from build123d import *

# Parameters (mm, degrees)
SKETCH_1_W               = 33.5
SKETCH_1_H               = 32
SKETCH_1_R               = 1.5
EXTRUDE_1_DEPTH          = 38
SKETCH_2_W               = 33
SKETCH_2_H               = 32
CUT_EXTRUDE_1_DEPTH      = 31
SKETCH_4_R               = 11.5
CUT_EXTRUDE_2_DEPTH      = 39
SKETCH_5_W               = 31
SKETCH_5_H               = 19
CUT_EXTRUDE_3_DEPTH      = 33.5
CUT_EXTRUDE_3_DEPTH_BACK = 11.5
SKETCH_8_W               = 38
SKETCH_8_H               = 32
EXTRUDE_3_DEPTH          = 4
EXTRUDE_4_DEPTH          = 9
SKETCH_11_W              = 8
SKETCH_11_H              = 1.5
CUT_EXTRUDE_4_DEPTH      = 10
FILLET_3_R               = 1
SKETCH_12_R              = 1.75
CUT_EXTRUDE_5_DEPTH      = 47.5
SKETCH_13_R              = 3.5
CUT_EXTRUDE_6_DEPTH      = 10
SKETCH_15_W              = 31.5
SKETCH_15_H              = 32
CUT_EXTRUDE_7_DEPTH      = 4
SKETCH_16_R              = 3
CUT_EXTRUDE_8_DEPTH      = 3
FILLET_4_R               = 5


with BuildPart() as part:
    # Эскиз1 → Бобышка-Вытянуть1 (new body)
    with BuildSketch(Plane.XY):
        with Locations((2.5, 0)):
            Rectangle(SKETCH_1_W, SKETCH_1_H)
        with Locations((10.25, -10)):
            Circle(SKETCH_1_R, mode=Mode.SUBTRACT)
        with Locations((-10.25, -10)):
            Circle(SKETCH_1_R, mode=Mode.SUBTRACT)
        with Locations((14.25, -10)):
            Circle(SKETCH_1_R, mode=Mode.SUBTRACT)
        with Locations((14.25, 10)):
            Circle(SKETCH_1_R, mode=Mode.SUBTRACT)
        with Locations((10.25, 10)):
            Circle(SKETCH_1_R, mode=Mode.SUBTRACT)
        with Locations((-10.25, 10)):
            Circle(SKETCH_1_R, mode=Mode.SUBTRACT)
    extrude(amount=-EXTRUDE_1_DEPTH)

    # Эскиз2 → Вырез-Вытянуть1 (cut)
    with BuildSketch(Plane.ZY.offset(14.25)):
        with Locations((-19, 0)):
            Rectangle(SKETCH_2_W, SKETCH_2_H)
    extrude(amount=-CUT_EXTRUDE_1_DEPTH, mode=Mode.SUBTRACT)

    # Эскиз4 → Вырез-Вытянуть2 (cut, through all)
    with BuildSketch(Plane(origin=(0, 0, -38), x_dir=(-1, 0, 0), z_dir=(0, 0, -1))):
        with Locations((19.35, 0)):
            Circle(SKETCH_4_R)
    extrude(amount=-CUT_EXTRUDE_2_DEPTH, mode=Mode.SUBTRACT)

    # Эскиз5 → Вырез-Вытянуть3 (cut, two sides)
    with BuildSketch(Plane.XY.offset(-35.5)) as cut_extrude_3_sk:
        with Locations((1.25, 0)):
            Rectangle(SKETCH_5_W, SKETCH_5_H)
    extrude(amount=CUT_EXTRUDE_3_DEPTH, mode=Mode.SUBTRACT)
    extrude(cut_extrude_3_sk.sketch, amount=-CUT_EXTRUDE_3_DEPTH_BACK, mode=Mode.SUBTRACT)

    # Эскиз8 → Бобышка-Вытянуть3 (add)
    with BuildSketch(Plane(origin=(19.25, 0, 0), x_dir=(0, 0, -1), z_dir=(1, 0, 0))):
        with Locations((19, 0)):
            Rectangle(SKETCH_8_W, SKETCH_8_H)
    extrude(amount=EXTRUDE_3_DEPTH)

    # Эскиз10 → Бобышка-Вытянуть4 (add)
    with BuildSketch(Plane(origin=(23.25, 0, 0), x_dir=(0, 0, -1), z_dir=(1, 0, 0))):
        with BuildLine():
            Line((38, 16), (0, 16))
            Line((0, 16), (-22.964648913, 10.720331419))
            ThreePointArc((-22.964648913, 10.720331419), (-31.5, 0), (-22.964648913, -10.720331419))
            Line((-22.964648913, -10.720331419), (0, -16))
            Line((0, -16), (38, -16))
            Line((38, -16), (38, 16))
        make_face()
    extrude(amount=EXTRUDE_4_DEPTH)

    # Эскиз11 → Вырез-Вытянуть4 (cut)
    with BuildSketch(Plane(origin=(0, 0, -38), x_dir=(-1, 0, 0), z_dir=(0, 0, -1))):
        with Locations((4.25, 10.25)):
            Rectangle(SKETCH_11_W, SKETCH_11_H)
        with Locations((4.25, -10.25)):
            Rectangle(SKETCH_11_W, SKETCH_11_H)
    extrude(amount=-CUT_EXTRUDE_4_DEPTH, mode=Mode.SUBTRACT)

    # Скругление3
    fillet_3_edges = [part.edges().sort_by_distance(p)[0] for p in [
        (-14.25, -16, -36.75),
        (-14.25, 16, -36.75),
        (-0.25, 11, -36.75),
        (-8.25, -11, -36.75),
        (-0.25, -11, -36.75),
        (-14.25, 16, -1.25),
        (-14.25, -16, -1.25),
        (-14.25, 10.307278981, -1.25),
        (-14.25, -10.307278981, -1.25),
        (-14.25, 10.307278981, -36.75),
        (-14.25, -10.307278981, -36.75),
    ]]
    fillet(fillet_3_edges, radius=FILLET_3_R)

    # Эскиз12 → Вырез-Вытянуть5 (cut, through all)
    with BuildSketch(Plane(origin=(32.25, 0, 0), x_dir=(0, 0, -1), z_dir=(1, 0, 0))):
        with Locations((-27.5, 0)):
            Circle(SKETCH_12_R)
        with Locations((-20.5, 7)):
            Circle(SKETCH_12_R)
        with Locations((-13.5, 0)):
            Circle(SKETCH_12_R)
        with Locations((-20.5, -7)):
            Circle(SKETCH_12_R)
    extrude(amount=-CUT_EXTRUDE_5_DEPTH, mode=Mode.SUBTRACT)

    # Эскиз13 → Вырез-Вытянуть6 (cut)
    with BuildSketch(Plane.ZY.offset(-23.25)):
        with Locations((20.5, 0)):
            Circle(SKETCH_13_R)
    extrude(amount=-CUT_EXTRUDE_6_DEPTH, mode=Mode.SUBTRACT)

    # Эскиз15 → Вырез-Вытянуть7 (cut)
    with BuildSketch(Plane.ZY.offset(-23.25)):
        with Locations((15.75, 0)):
            Rectangle(SKETCH_15_W, SKETCH_15_H)
    extrude(amount=-CUT_EXTRUDE_7_DEPTH, mode=Mode.SUBTRACT)

    # Эскиз16 → Вырез-Вытянуть8 (cut)
    with BuildSketch(Plane.ZY.offset(-27.25)):
        with Locations((20.5, 7)):
            Circle(SKETCH_16_R)
        with Locations((27.5, 0)):
            Circle(SKETCH_16_R)
        with Locations((20.5, -7)):
            Circle(SKETCH_16_R)
        with Locations((13.5, 0)):
            Circle(SKETCH_16_R)
    extrude(amount=-CUT_EXTRUDE_8_DEPTH, mode=Mode.SUBTRACT)

    # Скругление4
    fillet_4_edges = [part.edges().sort_by_distance(p)[0] for p in [
        (27.25, 0, 0),
    ]]
    fillet(fillet_4_edges, radius=FILLET_4_R)


solid = part.part
Read the model definition and answer for the solid it produces. Units are mm, in the model's axes. A direction names the side the tool comes from. Round coordinates to 2 decimals unless told otherwise and drop trailing zeros. Loops run counter-clockwise (first coordinate to the right, second up) from the corner with the lowest first, then second, coordinate; pieces in that order, holes last.
Q1. Determine the mould class of faces 1 (the face through (-7.85, 0.17, -0.99)), 2 (the face through (1, 13, -35.5)), 3 (the face through (14.2, -11.5, -36.7)) for opening direction X: released by +X, released by -X, zero draft, split by the parting line, or undercut.
Q2. Section A-A on x = 2.5 is taken. Write down the section's boundary in (y, z), and give its area (3 significant figures).
Q3. Each of these flat-tipped pins is pushed along its axis until it touches: pin 1 (2 mm diameter, centred on x = -9, y = 8, fed in from -Z); pin 2 (5 mm diameter, centred on x = -4, y = 12, fed in from +Z); pin 3 (2 mm diameter, centred on x = 26.5, z = 5.5, fed in from +Y). Where does it stop, or does it pass through?
Q4. Section D-D on y = 7 is taken. Write down the section's boundary in (x, z), and give its area (3 significant figures).
Q5. Section B-B on y = 0 is taken. Give the number of separate pieces and of enclosed holes in the cut face, and give its area (3 significant figures).
Q6. Section C-C on z = 20 is taken. Write down the section's boundary in (x, y), and give its area (3 significant figures).
Q7. Consider probe 1 along Z at (x, y) = (29.5, 0.5); probe 2 along X at (y, z) = (10, -37.2); probe 3 along Z at (x, y) = (16, 11). Determine where each line is inside the solid, lowest interval first.
Q8. Which of the six approach directions +Z, -Z, +X, -X, +Y, -Y give full straight-line access (tool end or side, diameter ignored) to faces 4 (the face through (-5, 11, -37)), 5 (the face through (4, -9.5, -37)), 6 (the face through (28.7, 0.1, 24.5))?
Output:
1. face 1: released by -X
1. face 2: zero draft
1. face 3: undercut
2. outline: (-16, -38) - (-9.5, -38) - (-9.5, -35.5) - (-16, -35.5) - close; (-16, -2.5) - (-9.5, -2.5) - (-9.5, -2) - (9.5, -2) - (9.5, -2.5) - (16, -2.5) - (16, 0) - (-16, 0) - close; (9.5, -38) - (16, -38) - (16, -35.5) - (9.5, -35.5) - close
2. area: 103 mm2
3. pin 1: stops at z = -2
3. pin 2: stops at z = 0
3. pin 3: stops at y = 14.89
4. outline: (-10.23, -2) - (16.75, -2) - (16.75, -38) - (32.25, -38) - (32.25, 18.75) - (30.25, 18.75) - (30.25, 17.5) - (27.25, 17.5) - (27.25, 5) arc R5 cw to (22.25, 0) - (-10.23, 0) - close; (27.25, 23.5) - (30.25, 23.5) - (30.25, 22.25) - (32.25, 22.25) - (32.25, 28.99) - (27.25, 28.99) - close
4. area: 768 mm2
5. separate pieces: 4
5. enclosed holes: 0
5. area: 716 mm2
6. outline: (27.25, -11.4) - (32.25, -11.4) - (32.25, -8.68) - (30.25, -8.68) - (30.25, -9.96) - (27.25, -9.96) - close; (27.25, -4.04) - (30.25, -4.04) - (30.25, -5.32) - (32.25, -5.32) - (32.25, -3.46) - (27.25, -3.46) - close; (27.25, 3.46) - (32.25, 3.46) - (32.25, 5.32) - (30.25, 5.32) - (30.25, 4.04) - (27.25, 4.04) - close; (27.25, 9.96) - (30.25, 9.96) - (30.25, 8.68) - (32.25, 8.68) - (32.25, 11.4) - (27.25, 11.4) - close
6. area: 30.5 mm2
7. probe 1: z = -38 to 10.54, 16.46 to 17.04, 23.96 to 24.54, 30.46 to 31.49
7. probe 2: x = -13.67 to -11.75, -8.75 to -8.25, -0.25 to 8.75, 11.75 to 12.75, 15.75 to 32.25
7. probe 3: z = -38 to -35.5, -2.5 to 0
8. face 4: -Z
8. face 5: -Z, -X
8. face 6: -X
